from build123d import *

# Parameters (mm, degrees)
F0_R     = 63.5
F1_DEPTH = 177.8
F2_R     = 25.4
F3_DEPTH = 76.2
F4_SIZE  = 25.4


with BuildPart() as f1:
    # F0 (on Right) → F1 (new body)
    with BuildSketch(Plane.YZ):
        Circle(F0_R)
    extrude(amount=F1_DEPTH)

    # F2 (on face) → F3 (cut)
    with BuildSketch(Plane(origin=(0, 0, 0), x_dir=(0, -1, 0), z_dir=(-1, 0, 0))):
        Circle(F2_R)
    extrude(amount=-F3_DEPTH, mode=Mode.SUBTRACT)

    # F4
    f4_edges = [f1.edges().sort_by_distance(p)[0] for p in [
        (0, -63.5, 0),
        (177.8, -63.5, 0),
    ]]
    chamfer(f4_edges, length=F4_SIZE)


solid = f1.part
Build history of the part. All positions in model axes, mm. Round coordinates to 2 decimals unless told otherwise and drop trailing zeros. Write each loop counter-clockwise with the first axis right and the second up, starting at its lowest first coordinate (ties: lowest second). Pieces come first, ordered by that corner, then holes. Notation, with made-up numbers: M 26,15 L 59,15 A21 ccw 59,24 Z; hole C 3.25,-20.75 d7. An arc over 180 degrees is marked long. Answer as a JSON object with one key per item and string values. Group by question number.
(1) Cut at C-C (x = 86). Give the cut face in (y, z).
(2) Drill centre lines: L1, parallel to Z at x = 39, y = 0; L2, parallel to Z at x = 25, y = 0; L3, parallel to Y at x = 57, z = 4. Where is each one in solid material? Low to high.
(3) Cut at D-D (x = 58.5). Give the cut face in (y, z).
(4) Flat gauge pins, fed straight in: pin 1 (3 mm diameter, centred on y = -14, z = -49, fed in from +X); pin 2 (10 mm diameter, centred on x = 138.5, y = 4, fed in from +Z); pin 3 (1 mm diameter, centred on x = 86, y = -46.5, fed in from -Z) (3 decimals). Where does each tip first touch, or does it go through?
(5) Cut at A-A (y = 0). Give the cut face in (x, z), and give its area (3 significant figures).
(6) Mould opens along Y. For faces 1 (the cylindrical face through (37.567, 5.506, -24.796)), 2 (the cylindrical face through (88.01, -13.77, -61.99)), 3 (the flat face through (76.2, 0, 0)), 4 (the flat face through (177.8, -1, 1)) say: pulls with the +Y half, pulls with the -Y half, needs draft (parallel to the pull), parting line crosses it, or undercut.
Responses:
{
 "1": {"outline": "C 0,0 d127"},
 "2": {"L1": "z = -63.5 to -25.4, 25.4 to 63.5", "L2": "z = -63.1 to -25.4, 25.4 to 63.1", "L3": "y = -63.37 to -25.08, 25.08 to 63.37"},
 "3": {"outline": "C 0,0 d127; hole C 0,0 d50.8"},
 "4": {"pin 1": "stops at x = 166.44", "pin 2": "stops at z = 63.5", "pin 3": "stops at z = -43.775"},
 "5": {"outline": "M 0,-38.1 L 25.4,-63.5 L 152.4,-63.5 L 177.8,-38.1 L 177.8,38.1 L 152.4,63.5 L 25.4,63.5 L 0,38.1 L 0,25.4 L 76.2,25.4 L 76.2,-25.4 L 0,-25.4 Z", "area": "17,400 mm2"},
 "6": {"face 1": "undercut", "face 2": "parting line crosses it", "face 3": "undercut", "face 4": "needs draft"}
}
